Could you check a few things on this drawing? It's one solid part, dimensions in mm from its lowest x, y, z. Round coordinates to 2 decimals unless told otherwise and drop trailing zeros. Write each loop counter-clockwise with the first axis right and the second up, starting at its lowest first coordinate (ties: lowest second). Pieces come first, ordered by that corner, then holes. Notation, with made-up numbers: (49.5, -26.75) -> (67.5, -26.75) arc R26 cw to (67.5, -4.75) -> close; hole circle Ø10 at (-39, 73). An arc over 180 degrees is marked (long way). Return JSON: item names as keys, results as strings.
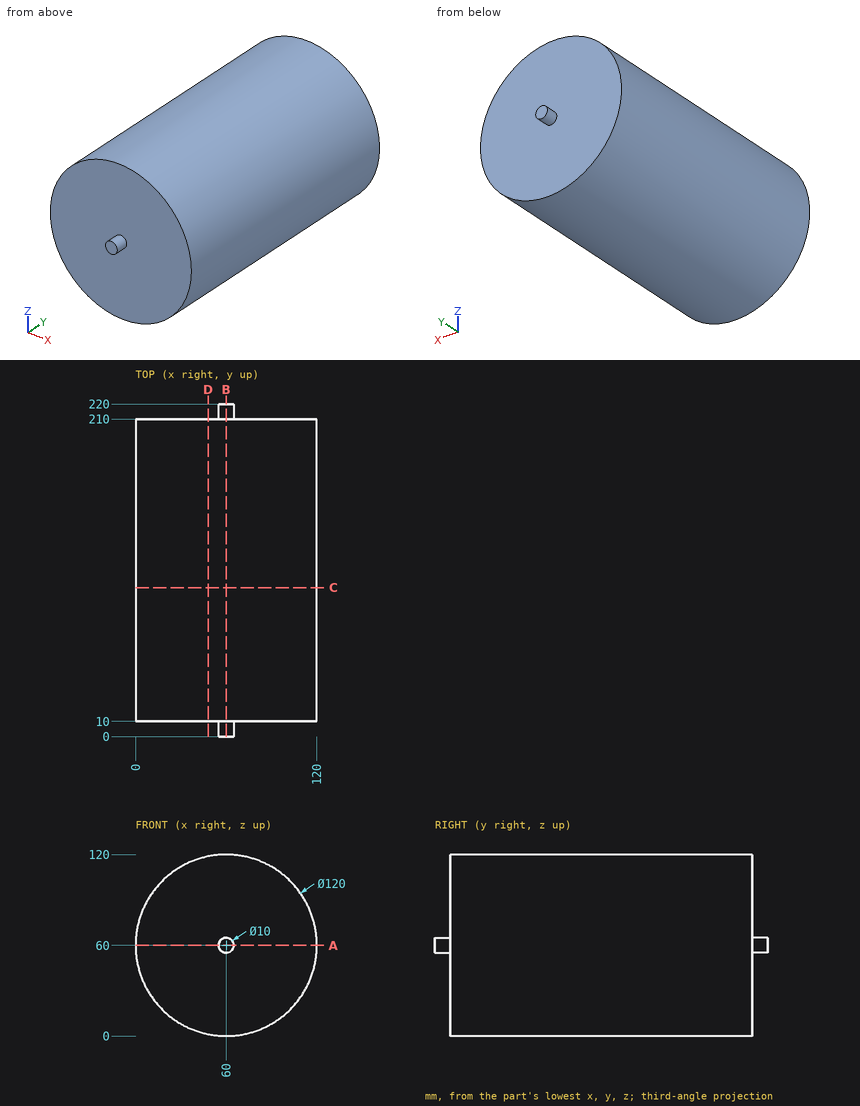
1) I want a section at D-D, the plane x = 48. Please give me the cut outline in (y, z), and give its area (3 significant figures).
Return value:
{"outline": "(10, 1.21) -> (210, 1.21) -> (210, 118.79) -> (10, 118.79) -> close", "area": "23,500 mm²"}
2) I want a section at A-A, the plane z = 60. Please give me the cut outline in (x, y).
Return value:
{"outline": "(0, 10) -> (55, 10) -> (55, 0) -> (65, 0) -> (65, 10) -> (120, 10) -> (120, 210) -> (65, 210) -> (65, 220) -> (55, 220) -> (55, 210) -> (0, 210) -> close"}
3) I want a section at B-B, the plane x = 60. Please give me the cut outline in (y, z).
Return value:
{"outline": "(0, 55) -> (10, 55) -> (10, 0) -> (210, 0) -> (210, 55) -> (220, 55) -> (220, 65) -> (210, 65) -> (210, 120) -> (10, 120) -> (10, 65) -> (0, 65) -> close"}
4) Will these pins go through, and if not, where does the flat tip stop? pin 1 Ø2 at (x, y) = (22.5, 28.5) entering from +Z; pin 2 Ø12 at (x, z) = (73.5, 37) entering from -Y; pin 3 Ø5 at (x, y) = (104.5, 93.5) entering from +Z.
Return value:
{"pin 1": "z = 107.62", "pin 2": "y = 10", "pin 3": "z = 102.85"}
5) I want a section at C-C, the plane y = 98.5. Please give me the cut outline in (x, z), and give its area (3 significant figures).
Return value:
{"outline": "circle Ø120 at (60, 60)", "area": "11,300 mm²"}
6) If I drill on probe 1 along Y at (x, z) = (79.5, 91.5); probe 2 along X at (y, z) = (181.5, 72); probe 3 along Z at (x, y) = (52, 197), over which ranges is the centre line in solid material (lowest first)? Write a range as [from, to].
Return value:
{"probe 1": "[10, 210]", "probe 2": "[1.21, 118.79]", "probe 3": "[0.54, 119.46]"}
